```python
from build123d import *

# Parameters (mm, degrees)
F0_W      = 45.5
F0_H      = 20.7
F0_R      = 0.75
F1_DEPTH  = 1.6
F2_R      = 8
F3_DEPTH  = 12.5
F2_W      = 10.5
F2_H      = 4.5
F4_DEPTH  = 3.3
F2_W_2    = 9.4
F2_H_2    = 2.3
F5_DEPTH  = 1.8
F7_DEPTH  = 2.75
F8_W      = 10.5
F8_H      = 2.5
F9_DEPTH  = 5
F10_W     = 10.5
F10_H     = 2.5
F11_DEPTH = 6.5


with BuildPart() as f1:
    # F0 (on Top) → F1 (new body)
    with BuildSketch(Plane.XY):
        Rectangle(F0_W, F0_H)
        with Locations((-21.3, -8.9)):
            Circle(F0_R, mode=Mode.SUBTRACT)
        with Locations((21.3, -8.9)):
            Circle(F0_R, mode=Mode.SUBTRACT)
        with Locations((-21.3, 8.9)):
            Circle(F0_R, mode=Mode.SUBTRACT)
        with Locations((21.3, 8.9)):
            Circle(F0_R, mode=Mode.SUBTRACT)
    extrude(amount=F1_DEPTH)

    # F2 (on face) → F3 (join)
    with BuildSketch(Plane.XY.offset(1.6)):
        with Locations((-13.15, 0)):
            Circle(F2_R)
        with Locations((13.15, 0)):
            Circle(F2_R)
    extrude(amount=F3_DEPTH)

    # F2 (on face) → F4 (join)
    with BuildSketch(Plane.XY.offset(1.6)):
        with Locations((0, 7.35)):
            Rectangle(F2_W, F2_H)
    extrude(amount=F4_DEPTH)

    # F2 (on face) → F5 (join)
    with BuildSketch(Plane.XY.offset(1.6)):
        with Locations((0, -8.7)):
            Rectangle(F2_W_2, F2_H_2)
    extrude(amount=F5_DEPTH)

    # F6 (on face) → F7 (join)
    with BuildSketch(Plane(origin=(0, 0, 0), x_dir=(1, 0, 0), z_dir=(0, 0, -1))):
        Polygon((-20.25, -7.45), (-20.25, -10.35), (20.25, -10.35), (20.25, -7.45), (22.75, -7.45), (22.75, 7.45), (20.25, 7.45), (20.25, 10.35), (-20.25, 10.35), (-20.25, 7.45), (-22.75, 7.45), (-22.75, -7.45), align=None)
    extrude(amount=F7_DEPTH)

    # F8 (on face) → F9 (join)
    with BuildSketch(Plane(origin=(0, 0, -2.75), x_dir=(1, 0, 0), z_dir=(0, 0, -1))):
        with Locations((0, 8.85)):
            Rectangle(F8_W, F8_H)
    extrude(amount=F9_DEPTH)

    # F10 (on face) → F11 (join)
    with BuildSketch(Plane.XZ.offset(10.1)):
        with Locations((0, -6.5)):
            Rectangle(F10_W, F10_H)
    extrude(amount=F11_DEPTH)


solid = f1.part
```
Check sheet for the modelled part. Datum: model origin and axes. Units: mm. A direction names the side the tool comes from. Give positions to 0.01 mm unless a question says otherwise; leave off trailing zeros. Write each loop counter-clockwise with the first axis right and the second up, starting at its lowest first coordinate (ties: lowest second). Pieces come first, ordered by that corner, then holes. Notation, with made-up numbers: (-37.5, 58.25) - (-2.5, 58.25) arc R15 cw to (-2.5, 75.25) - close; hole circle Ø6 at (36, 44.25). An arc over 180 degrees is marked (long way). Answer as a JSON object with one key per item and string values. Group by question number.
1) Depth check by flat-ended pin: P1, Ø5, axis at x = 2, z = -1, coming from the -Y side; P2, Ø5, axis at x = -0.5, z = 6, coming from the -Y side; P3, Ø6, axis at x = -13.5, y = 4, coming from the -Z side; P4, Ø1.4, axis at x = -21.3, y = -8.9, coming from the +Z side. Enter the tip coordinate at first touch or a pass-through.
2) Thickness scan on probe 1 along Y at (x, z) = (-21.3, 0.85); probe 2 along Z at (x, y) = (-19.5, 3.5); probe 3 along Z at (x, y) = (20, 9). Record the ranges inside material, lowest first. Write a range as from..to.
3) Sectioned sample at B-B (x = -13.15). Record the cut outline in (y, z), then the cut area to 3 significant figures.
4) Sectioned sample at C-C (z = 8.5). Record the cut outline in (x, y), then the cut area to 3 significant figures.
5) Access from +Z, -Z, +X, -X, +Y, -Y to the whole of each face (thin tool, end or side, straight path). Record for faces 1 (the face through (0, 5.1, 3)), 2 (the face through (22, -8, 0)), 3 (the face through (22, 10, 0)).
6) Release check for a two-part mould opening along X. For faces 4 (the face through (-5.25, -11, -6)), 5 (the face through (0, -10.35, -1)), 6 (the face through (4.7, -9, 2)) record: pulls with the +X half, pulls with the -X half, needs draft (parallel to the pull), parting line crosses it, or undercut.
7) Sectioned sample at A-A (y = 8.9). Record the cut outline in (x, z), then the cut area to 3 significant figures.
8) Sectioned sample at D-D (y = 0). Record the cut outline in (x, z).
Geometry results:
{
 "1": {"P1": "stops at y = -10.35", "P2": "stops at y = 5.1", "P3": "stops at z = -2.75", "P4": "passes through"},
 "2": {"probe 1": "y = -10.35..-9.65, -8.15..8.15, 9.65..10.35", "probe 2": "z = -2.75..14.1", "probe 3": "z = -2.75..1.6"},
 "3": {"outline": "(-10.35, -2.75) - (10.35, -2.75) - (10.35, 1.6) - (8, 1.6) - (8, 14.1) - (-8, 14.1) - (-8, 1.6) - (-10.35, 1.6) - close", "area": "290 mm^2"},
 "4": {"outline": "circle Ø16 at (-13.15, 0); circle Ø16 at (13.15, 0)", "area": "402 mm^2"},
 "5": {"face 1": "+Z", "face 2": "-Z, +X, -Y", "face 3": "-Z, +X, +Y"},
 "6": {"face 4": "pulls with the -X half", "face 5": "needs draft", "face 6": "undercut"},
 "7": {"outline": "(-22.75, 0) - (-22.05, 0) - (-22.05, 1.6) - (-22.75, 1.6) - close; (-20.55, 0) - (-20.25, 0) - (-20.25, -2.75) - (20.25, -2.75) - (20.25, 0) - (20.55, 0) - (20.55, 1.6) - (5.25, 1.6) - (5.25, 4.9) - (-5.25, 4.9) - (-5.25, 1.6) - (-20.55, 1.6) - close; (22.05, 0) - (22.75, 0) - (22.75, 1.6) - (22.05, 1.6) - close", "area": "214 mm^2"},
 "8": {"outline": "(-22.75, -2.75) - (22.75, -2.75) - (22.75, 1.6) - (21.15, 1.6) - (21.15, 14.1) - (5.15, 14.1) - (5.15, 1.6) - (-5.15, 1.6) - (-5.15, 14.1) - (-21.15, 14.1) - (-21.15, 1.6) - (-22.75, 1.6) - close"}
}
